Read the model definition and answer for the solid it produces. Units are mm, in the model's axes. A direction names the side the tool comes from. Coordinates: 2 decimals unless noted, no trailing zeros. Write each loop counter-clockwise with the first axis right and the second up, starting at its lowest first coordinate (ties: lowest second). Pieces come first, ordered by that corner, then holes.
(1) Section D-D on z = -38 is taken. State how many separate pieces and enclosed holes the cut face has, then the cut area to 3 significant figures.
(2) Section B-B on y = 623.5 is taken. Write down the section's boundary in (x, z).
(3) Which of the six approach directions +Z, -Z, +X, -X, +Y, -Y give full straight-line access (tool end or side, diameter ignored) to faces 4 (the flat face through (199, -374, -377.825)), 5 (the flat face through (533.4, -348, 5)), 6 (the flat face through (-304.8, -397, -378))?
(4) Section C-C on x = -340 is taken. Write down the section's boundary in (y, z) (3 decimals), then the cut area to 3 significant figures.
(5) Given pin 1 (0.8 mm diameter, centred on x = 339, z = 380, fed in from -Y); pin 2 (1 mm diameter, centred on y = 284.5, z = -292, fed in from -X); pin 3 (3 mm diameter, centred on x = -335, z = 151, fed in from -Y), each flat-ended and moving along its own axis, determine where each tip first touches the part or whether it passes through.
(6) Section A-A on z = 285 is taken. Write down the section's boundary in (x, y) (3 decimals).
(7) Find the intervals of material crossed by probe 1 along Y at (x, z) = (-366.5, -29.5) (3 decimals); probe 2 along X at (y, z) = (-665.5, 291) (3 decimals); probe 3 along Z at (x, y) = (-19, -407) (3 decimals), in increasing order.
(8) The mould has two halves that part along Z. Classify faces 1 (the flat face through (-408, -374, -377.825)), 2 (the flat face through (-101.6, -390, -378)), 3 (the flat face through (305, 384, 6.35)): +Z half, -Z half, draft (parallel to the pull), parting line (faces both ways), or undercut.
from build123d import *

# Parameters (mm, degrees)
SKETCH1_W            = 1066.8
SKETCH1_H            = 762
BOSS_EXTRUDE1_DEPTH  = 2.54
SKETCH2_W            = 203.2
SKETCH2_H            = 139.7
CUT_EXTRUDE1_DEPTH   = 656.50210648
SKETCH3_W            = 25.4
SKETCH3_H            = 25.4
BOSS_EXTRUDE2_DEPTH  = 762
SKETCH4_W            = 406.4
SKETCH4_H            = 381
BOSS_EXTRUDE3_DEPTH  = 508
SKETCH5_R            = 12.7
BOSS_EXTRUDE4_DEPTH  = 12.7
SKETCH6_W            = 3.94766101
SKETCH6_H            = 20.265990969
BOSS_EXTRUDE5_DEPTH  = 3.175
FILLET1_R            = 2.54
SKETCH7_W            = 196.85
SKETCH7_H            = 101.6
BOSS_EXTRUDE6_DEPTH  = 6.35
FILLET2_R            = 2.54
SKETCH8_W            = 2.54
SKETCH8_H            = 25.4
SKETCH8_W_2          = 203.2
SKETCH8_H_2          = 2.54
SKETCH8_W_3          = 406.4
BOSS_EXTRUDE7_DEPTH  = 759.46
SKETCH9_W            = 1066.8
SKETCH9_H            = 762
BOSS_EXTRUDE8_DEPTH  = 3.175
SKETCH11_W           = 1016
SKETCH11_H           = 3.175
SKETCH11_W_2         = 3.175
SKETCH11_H_2         = 711.2
SKETCH11_W_3         = 203.2
SKETCH11_W_4         = 609.6
BOSS_EXTRUDE10_DEPTH = 759.46
CUT_EXTRUDE3_REACH   = 1366.534
SKETCH12_W           = 254
SKETCH12_H           = 25.4
CUT_EXTRUDE4_REACH   = 1206.43
SKETCH13_W           = 254
SKETCH13_H           = 25.4
SKETCH14_W           = 495.3
SKETCH14_H           = 706.721299259
SKETCH14_W_2         = 490.22
SKETCH14_H_2         = 701.641299259
CUT_EXTRUDE5_DEPTH   = 2.54


with BuildPart() as part:
    # Sketch1 → Boss-Extrude1 (new body)
    with BuildSketch(Plane(origin=(0, 0, 0), x_dir=(1, 0, 0), z_dir=(0, 1, 0))):
        Rectangle(SKETCH1_W, SKETCH1_H)
    extrude(amount=BOSS_EXTRUDE1_DEPTH)

    # Sketch2 → Cut-Extrude1 (cut, through all)
    with BuildSketch(Plane(origin=(0, 2.54, 0), x_dir=(1, 0, 0), z_dir=(0, 1, 0))):
        with Locations((-203.2, 311.15)):
            Rectangle(SKETCH2_W, SKETCH2_H)
    extrude(amount=-CUT_EXTRUDE1_DEPTH, mode=Mode.SUBTRACT)

    # Sketch3 → Boss-Extrude2 (add)
    with BuildSketch(Plane.XZ):
        with Locations((-520.7, 368.3)):
            Rectangle(SKETCH3_W, SKETCH3_H)
        with Locations((520.7, 368.3)):
            Rectangle(SKETCH3_W, SKETCH3_H)
        with Locations((520.7, -368.3)):
            Rectangle(SKETCH3_W, SKETCH3_H)
        with Locations((-520.7, -368.3)):
            Rectangle(SKETCH3_W, SKETCH3_H)
    extrude(amount=BOSS_EXTRUDE2_DEPTH)

    # Sketch4 → Boss-Extrude3 (add)
    with BuildSketch(Plane(origin=(0, 2.54, 0), x_dir=(1, 0, 0), z_dir=(0, 1, 0))):
        with Locations((304.8, 190.5)):
            Rectangle(SKETCH4_W, SKETCH4_H)
    extrude(amount=BOSS_EXTRUDE3_DEPTH)

    # Sketch5 → Boss-Extrude4 (add)
    with BuildSketch(Plane.XY):
        with Locations(Location((203.2, 256.54, 0), (0, 0, 180))):
            Circle(SKETCH5_R)
        with Locations(Location((304.8, 256.54, 0), (0, 0, 180))):
            Circle(SKETCH5_R)
        with Locations(Location((406.4, 256.54, 0), (0, 0, 180))):
            Circle(SKETCH5_R)
    extrude(amount=BOSS_EXTRUDE4_DEPTH)

    # Sketch6 → Boss-Extrude5 (add)
    with BuildSketch(Plane.XY.offset(12.7)):
        with Locations((406.4, 256.600571442)):
            Rectangle(SKETCH6_W, SKETCH6_H)
    extrude(amount=BOSS_EXTRUDE5_DEPTH)

    # Fillet1
    fillet1_edges = [part.edges().sort_by_distance(p)[0] for p in [
        (406.4, 266.733566926, 15.875),
    ]]
    fillet(fillet1_edges, radius=FILLET1_R)

    # Sketch7 → Boss-Extrude6 (add)
    with BuildSketch(Plane.XY):
        with Locations((306.763896215, 383.54)):
            Rectangle(SKETCH7_W, SKETCH7_H)
    extrude(amount=BOSS_EXTRUDE6_DEPTH)

    # Fillet2
    fillet2_edges = [part.edges().sort_by_distance(p)[0] for p in [
        (208.338896215, 383.54, 6.35),
        (306.763896215, 332.74, 6.35),
        (405.188896215, 383.54, 6.35),
        (306.763896215, 434.34, 6.35),
    ]]
    fillet(fillet2_edges, radius=FILLET2_R)

    # Sketch8 → Boss-Extrude7 (add)
    with BuildSketch(Plane(origin=(0, 2.54, 0), x_dir=(1, 0, 0), z_dir=(0, 1, 0))):
        Polygon((-304.8, 381), (-533.4, 381), (-533.4, 378.46), (-530.86, 378.46), (-304.8, 378.46), align=None)
        with Locations((-532.13, 365.76)):
            Rectangle(SKETCH8_W, SKETCH8_H)
        Polygon((530.86, 378.46), (533.4, 378.46), (533.4, 381), (508, 381), (508, 378.46), align=None)
        with Locations((532.13, 365.76)):
            Rectangle(SKETCH8_W, SKETCH8_H)
        with Locations((0, 379.73)):
            Rectangle(SKETCH8_W_2, SKETCH8_H_2)
        Polygon((508, -378.46), (508, -381), (533.4, -381), (533.4, -378.46), (530.86, -378.46), align=None)
        with Locations((532.13, -365.76)):
            Rectangle(SKETCH8_W, SKETCH8_H)
        with Locations((-532.13, -365.76)):
            Rectangle(SKETCH8_W, SKETCH8_H)
        Polygon((-530.86, -378.46), (-533.4, -378.46), (-533.4, -381), (-508, -381), (-508, -378.46), align=None)
        with Locations((304.8, 379.73)):
            Rectangle(SKETCH8_W_3, SKETCH8_H_2)
    extrude(amount=BOSS_EXTRUDE7_DEPTH)

    # Sketch9 → Boss-Extrude8 (add)
    with BuildSketch(Plane(origin=(0, 762, 0), x_dir=(1, 0, 0), z_dir=(0, 1, 0))):
        Rectangle(SKETCH9_W, SKETCH9_H)
    extrude(amount=BOSS_EXTRUDE8_DEPTH)

    # Sketch11 → Boss-Extrude10 (add)
    with BuildSketch(Plane.XZ):
        with Locations((0, 379.4125)):
            Rectangle(SKETCH11_W, SKETCH11_H)
        with Locations((531.8125, 0)):
            Rectangle(SKETCH11_W_2, SKETCH11_H_2)
        with Locations((-531.8125, 0)):
            Rectangle(SKETCH11_W_2, SKETCH11_H_2)
        with Locations((-406.4, -379.4125)):
            Rectangle(SKETCH11_W_3, SKETCH11_H)
        with Locations((203.2, -379.4125)):
            Rectangle(SKETCH11_W_4, SKETCH11_H)
    extrude(amount=BOSS_EXTRUDE10_DEPTH)

    # Sketch12 → Cut-Extrude3 (cut, up to next)
    with BuildSketch(Plane.ZY.offset(-530.225), mode=Mode.PRIVATE) as cut_extrude3_sk1:
        with Locations((-127, -317.5)):
            Rectangle(SKETCH12_W, SKETCH12_H)
    cut_extrude3_tool1 = extrude(cut_extrude3_sk1.sketch, amount=-CUT_EXTRUDE3_REACH, mode=Mode.PRIVATE) & part.part
    # Sketch12 → Cut-Extrude3 (cut, up to next)
    with BuildSketch(Plane.ZY.offset(-530.225), mode=Mode.PRIVATE) as cut_extrude3_sk2:
        with Locations((-127, -393.7)):
            Rectangle(SKETCH12_W, SKETCH12_H)
    cut_extrude3_tool2 = extrude(cut_extrude3_sk2.sketch, amount=-CUT_EXTRUDE3_REACH, mode=Mode.PRIVATE) & part.part
    # Sketch12 → Cut-Extrude3 (cut, up to next)
    with BuildSketch(Plane.ZY.offset(-530.225), mode=Mode.PRIVATE) as cut_extrude3_sk3:
        with Locations((-127, -469.9)):
            Rectangle(SKETCH12_W, SKETCH12_H)
    cut_extrude3_tool3 = extrude(cut_extrude3_sk3.sketch, amount=-CUT_EXTRUDE3_REACH, mode=Mode.PRIVATE) & part.part
    # Sketch12 → Cut-Extrude3 (cut, up to next)
    with BuildSketch(Plane.ZY.offset(-530.225), mode=Mode.PRIVATE) as cut_extrude3_sk4:
        with Locations((-127, -546.1)):
            Rectangle(SKETCH12_W, SKETCH12_H)
    cut_extrude3_tool4 = extrude(cut_extrude3_sk4.sketch, amount=-CUT_EXTRUDE3_REACH, mode=Mode.PRIVATE) & part.part
    add(cut_extrude3_tool1.solids().sort_by_distance((530.225, -317.5, -127))[0], mode=Mode.SUBTRACT)
    add(cut_extrude3_tool2.solids().sort_by_distance((530.225, -393.7, -127))[0], mode=Mode.SUBTRACT)
    add(cut_extrude3_tool3.solids().sort_by_distance((530.225, -469.9, -127))[0], mode=Mode.SUBTRACT)
    add(cut_extrude3_tool4.solids().sort_by_distance((530.225, -546.1, -127))[0], mode=Mode.SUBTRACT)

    # Sketch13 → Cut-Extrude4 (cut, up to next)
    with BuildSketch(Plane(origin=(0, 0, -381), x_dir=(-1, 0, 0), z_dir=(0, 0, -1)), mode=Mode.PRIVATE) as cut_extrude4_sk1:
        with Locations((-279.4, -317.5)):
            Rectangle(SKETCH13_W, SKETCH13_H)
    cut_extrude4_tool1 = extrude(cut_extrude4_sk1.sketch, amount=-CUT_EXTRUDE4_REACH, mode=Mode.PRIVATE) & part.part
    # Sketch13 → Cut-Extrude4 (cut, up to next)
    with BuildSketch(Plane(origin=(0, 0, -381), x_dir=(-1, 0, 0), z_dir=(0, 0, -1)), mode=Mode.PRIVATE) as cut_extrude4_sk2:
        with Locations((-279.4, -393.7)):
            Rectangle(SKETCH13_W, SKETCH13_H)
    cut_extrude4_tool2 = extrude(cut_extrude4_sk2.sketch, amount=-CUT_EXTRUDE4_REACH, mode=Mode.PRIVATE) & part.part
    # Sketch13 → Cut-Extrude4 (cut, up to next)
    with BuildSketch(Plane(origin=(0, 0, -381), x_dir=(-1, 0, 0), z_dir=(0, 0, -1)), mode=Mode.PRIVATE) as cut_extrude4_sk3:
        with Locations((-279.4, -469.9)):
            Rectangle(SKETCH13_W, SKETCH13_H)
    cut_extrude4_tool3 = extrude(cut_extrude4_sk3.sketch, amount=-CUT_EXTRUDE4_REACH, mode=Mode.PRIVATE) & part.part
    # Sketch13 → Cut-Extrude4 (cut, up to next)
    with BuildSketch(Plane(origin=(0, 0, -381), x_dir=(-1, 0, 0), z_dir=(0, 0, -1)), mode=Mode.PRIVATE) as cut_extrude4_sk4:
        with Locations((-279.4, -546.1)):
            Rectangle(SKETCH13_W, SKETCH13_H)
    cut_extrude4_tool4 = extrude(cut_extrude4_sk4.sketch, amount=-CUT_EXTRUDE4_REACH, mode=Mode.PRIVATE) & part.part
    add(cut_extrude4_tool1.solids().sort_by_distance((279.4, -317.5, -381))[0], mode=Mode.SUBTRACT)
    add(cut_extrude4_tool2.solids().sort_by_distance((279.4, -393.7, -381))[0], mode=Mode.SUBTRACT)
    add(cut_extrude4_tool3.solids().sort_by_distance((279.4, -469.9, -381))[0], mode=Mode.SUBTRACT)
    add(cut_extrude4_tool4.solids().sort_by_distance((279.4, -546.1, -381))[0], mode=Mode.SUBTRACT)

    # Sketch14 → Cut-Extrude5 (cut)
    # profile 1 of 2: a face of its own
    with BuildSketch(Plane.XY.offset(381)):
        with Locations((-260.35, -379.817122747)):
            Rectangle(SKETCH14_W, SKETCH14_H)
        with Locations((-260.35, -379.817122748)):
            Rectangle(SKETCH14_W_2, SKETCH14_H_2, mode=Mode.SUBTRACT)
    # profile 2 of 2: a face of its own
    with BuildSketch(Plane.XY.offset(381)):
        with Locations((260.35, -379.817122747)):
            Rectangle(SKETCH14_W, SKETCH14_H)
        with Locations((260.35, -379.817122748)):
            Rectangle(SKETCH14_W_2, SKETCH14_H_2, mode=Mode.SUBTRACT)
    extrude(amount=-CUT_EXTRUDE5_DEPTH, mode=Mode.SUBTRACT)


solid = part.part
Response:
1. separate pieces: 6
1. enclosed holes: 0
1. area: 217,000 mm2
2. outline: (-533.4, -381) - (-304.8, -381) - (-304.8, -378.46) - (-530.86, -378.46) - (-530.86, -353.06) - (-533.4, -353.06) - close; (-533.4, 353.06) - (-530.86, 353.06) - (-530.86, 378.46) - (-508, 378.46) - (-508, 381) - (-533.4, 381) - close; (-101.6, -381) - (533.4, -381) - (533.4, -353.06) - (530.86, -353.06) - (530.86, -378.46) - (-101.6, -378.46) - close; (508, 378.46) - (530.86, 378.46) - (530.86, 353.06) - (533.4, 353.06) - (533.4, 381) - (508, 381) - close
3. face 4: -Y
3. face 5: +Z, -Z, +X, +Y, -Y
3. face 6: -Z, -Y
4. outline: (-759.46, -381) - (765.175, -381) - (765.175, 381) - (762, 381) - (762, -378.46) - (2.54, -378.46) - (2.54, 381) - (-26.456, 381) - (-26.456, 378.46) - (-28.996, 378.46) - (-28.996, 381) - (-730.638, 381) - (-730.638, 378.46) - (-733.178, 378.46) - (-733.178, 381) - (-759.46, 381) - (-759.46, 377.825) - (0, 377.825) - (0, -377.825) - (-759.46, -377.825) - close
4. area: 11,100 mm2
5. pin 1: stops at y = -759.46
5. pin 2: stops at x = 101.6
5. pin 3: stops at y = 0
6. outline: (-533.4, -759.46) - (-530.225, -759.46) - (-530.225, 0) - (530.225, 0) - (530.225, -759.46) - (533.4, -759.46) - (533.4, 2.54) - (-533.4, 2.54) - close; (-533.4, 762) - (533.4, 762) - (533.4, 765.175) - (-533.4, 765.175) - close
7. probe 1: y = 0 to 2.54, 762 to 765.175
7. probe 2: x = -533.4 to -530.225, 530.225 to 533.4
7. probe 3: z = -381 to -377.825, 377.825 to 381
8. face 1: undercut
8. face 2: draft
8. face 3: +Z half
